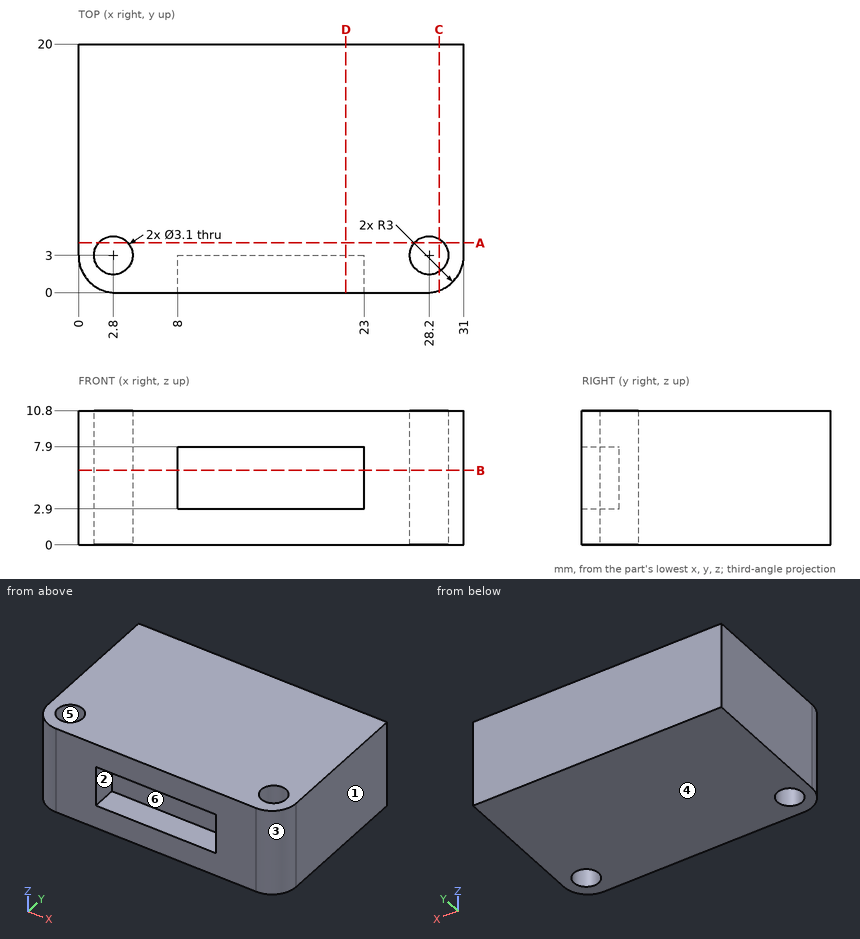
For this review, use the dimensioned drawing (mm, ordinates from the lowest corner) and the shaded views. A direction names the side the tool comes from. Round coordinates to 2 decimals unless told otherwise and drop trailing zeros. Order: outer loops, then holes, each group sorted by start corner. A loop starts at its lowest first (then second) coordinate and runs counter-clockwise, first axis right, second up. Notation, with made-up numbers: (43, -9) -> (64, -9) arc R35 cw to (64, 23) -> close; hole circle Ø11 at (16.5, 5.5). An arc over 180 degrees is marked (long way). One line per item, written item: value. Start each with the question number.
Q1. Wall thickness on line 1 (Y direction, x = 28.2, z = 4); line 2 (X direction, y = 2.5, z = 6); line 3 (X direction, y = 2.75, z = 8): over which ranges is each line inside the solid? List them lowest first.
Q2. Machinability: for the marked faces 1 and 2, which of the approach directions +Z, -Z, +X, -X, +Y, -Y give a long, thin tool a straight path to every point of the face, cutting with its end or side? Answer none if there is none.
Q3. Take a section at B-B (z = 6). Write out the cut boundary in (x, y).
Q4. Take a section at A-A (y = 4). Write out the cut boundary in (x, z).
Q5. Take a section at C-C (x = 29). Write out the cut boundary in (y, z).
Q6. Take a section at D-D (x = 21.5). Write out the cut boundary in (y, z).
Q7. Clearance check with flat-ended pins moving along their axes: pin 1 Ø1.5 at (x, z) = (15.5, 6.5) entering from -Y; pin 2 Ø0.9 at (y, z) = (1.5, 6.5) entering from -X. State where each tip first meets the part, or that it passes through.
Q8. Mouldability with a two-part tool opening along X and no side actions: class the marked faces 3, 4, 5 and 6 as released by +X, released by -X, zero draft, split by the parting line, or undercut.
Reported:
1. line 1: y = 0.01 to 1.45, 4.55 to 20
1. line 2: x = 0.04 to 1.33, 4.27 to 8, 23 to 26.73, 29.67 to 30.96
1. line 3: x = 0.01 to 1.27, 4.33 to 26.67, 29.73 to 30.99
2. face 1: +Z, -Z, +X, +Y, -Y
2. face 2: -Y
3. outline: (0, 3) arc R3 ccw to (3, 0) -> (8, 0) -> (8, 3) -> (23, 3) -> (23, 0) -> (28, 0) arc R3 ccw to (31, 3) -> (31, 20) -> (0, 20) -> close; hole circle Ø3.1 at (2.8, 3); hole circle Ø3.1 at (28.2, 3)
4. outline: (0, 0) -> (1.62, 0) -> (1.62, 10.8) -> (0, 10.8) -> close; (3.98, 0) -> (27.02, 0) -> (27.02, 10.8) -> (3.98, 10.8) -> close; (29.38, 0) -> (31, 0) -> (31, 10.8) -> (29.38, 10.8) -> close
5. outline: (0.17, 0) -> (1.67, 0) -> (1.67, 10.8) -> (0.17, 10.8) -> close; (4.33, 0) -> (20, 0) -> (20, 10.8) -> (4.33, 10.8) -> close
6. outline: (0, 0) -> (20, 0) -> (20, 10.8) -> (0, 10.8) -> (0, 7.9) -> (3, 7.9) -> (3, 2.9) -> (0, 2.9) -> close
7. pin 1: stops at y = 3
7. pin 2: stops at x = 0.19
8. face 3: released by +X
8. face 4: zero draft
8. face 5: undercut
8. face 6: undercut
